Read the model definition and answer for the solid it produces. Units are mm, in the model's axes. Coordinates: 2 decimals unless noted, no trailing zeros. Write each loop counter-clockwise with the first axis right and the second up, starting at its lowest first coordinate (ties: lowest second). Pieces come first, ordered by that corner, then holes.
(1) Given pin 1 (6.5 mm diameter, centred on y = 8, z = 299, fed in from -X); pin 2 (4 mm diameter, centred on x = 314.5, y = 8.5, fed in from +Z); pin 3 (5 mm diameter, centred on y = 7.5, z = 7.5, fed in from -X), each flat-ended and moving along its own axis, determine where each tip first touches the part or whether it passes through.
(2) Section C-C on z = 265.5 is taken. Write down the section's boundary in (x, y).
(3) Section A-A on z = 37 is taken. Write down the section's boundary in (x, y), then the cut area to 3 significant figures.
(4) Find the intervals of material crossed by probe 1 along X at (y, z) = (1.5, -307.5); probe 2 along Z at (x, y) = (-57.5, 7.5); probe 3 along Z at (x, y) = (46, 6.25), in increasing order.
(5) The mould has two halves that part along Z. Classify faces 1 (the cylindrical face through (-253.76, 6.26, -11.08)), 2 (the flat face through (234, 12.7, -103)), 3 (the cylindrical face through (76.975, 6.261, -332.519)): +Z half, -Z half, draft (parallel to the pull), parting line (faces both ways), or undercut.
(6) Section B-B on x = -170 is taken. Write down the section's boundary in (y, z), then the cut area to 3 significant figures.
from build123d import *

# Parameters (mm, degrees)
BOSS_EXTRUDE1_DEPTH                          = 12.7
M8X1_25_TAPPED_HOLE1_FOR_LOWERING_D          = 6.8
M8_CLEARANCE_HOLE1_FOR_SPACER_BLOCK_D        = 9
M8_CLEARANCE_HOLE2_FOR_CLAMP_TIGHTENIN_D     = 9
M8_CLEARANCE_HOLE2_FOR_CLAMP_TIGHTENIN_DEPTH = 20
M8X1_25_TAPPED_HOLE2_FOR_CLAMP_TIGHTEN_D     = 6.8
BOSS_EXTRUDE2_START                          = -12.7
BOSS_EXTRUDE2_HANDLES_DEPTH                  = 12.7


with BuildPart() as part:
    # Sketch1 → Boss-Extrude1 (new body)
    with BuildSketch(Plane(origin=(0, 0, 0), x_dir=(1, 0, 0), z_dir=(0, 1, 0))):
        with BuildLine():
            Line((275.144331903, 6), (253.92912397, 6))
            ThreePointArc((253.92912397, 6), (-254, 0), (253.92912397, -6))
            Line((253.92912397, -6), (275.067203981, -6))
            Line((275.067203981, -6), (336.321934193, -6))
            Line((336.321934193, -6), (336.321934193, -26))
            Line((336.321934193, -26), (286.321934193, -26))
            ThreePointArc((286.321934193, -26), (-287.5, 0), (286.321934193, 26))
            Line((286.321934193, 26), (336.321934193, 26))
            Line((336.321934193, 26), (336.321934193, 6))
            Line((336.321934193, 6), (275.144331903, 6))
        make_face()
    extrude(amount=BOSS_EXTRUDE1_DEPTH)

    # M8x1.25 Tapped Hole1 - For Lowering (through all)
    with Locations(Plane(origin=(0, 12.7, 0), x_dir=(1, 0, 0), z_dir=(0, 1, 0))):
        with Locations((135.375, -234.476378075), (-270.75, 0), (135.375, 234.476378075)):
            Hole(M8X1_25_TAPPED_HOLE1_FOR_LOWERING_D / 2)

    # M8 Clearance Hole1 - For Spacer Block (through all)
    with Locations(Plane(origin=(0, 12.7, 0), x_dir=(1, 0, 0), z_dir=(0, 1, 0))):
        with Locations((0, 270.75), (234.476378075, -135.375), (-234.476378075, -135.375)):
            Hole(M8_CLEARANCE_HOLE1_FOR_SPACER_BLOCK_D / 2)

    # M8 Clearance Hole2 - For Clamp Tightening
    with Locations(Plane(origin=(0, 0, -26), x_dir=(-1, 0, 0), z_dir=(0, 0, -1))):
        with Locations((-311.321934193, 6.35)):
            Hole(M8_CLEARANCE_HOLE2_FOR_CLAMP_TIGHTENIN_D / 2, depth=M8_CLEARANCE_HOLE2_FOR_CLAMP_TIGHTENIN_DEPTH)

    # M8x1.25 Tapped Hole2 - For Clamp Tightening (through all)
    with Locations(Plane.XY.offset(26)):
        with Locations((311.321934193, 6.35)):
            Hole(M8X1_25_TAPPED_HOLE2_FOR_CLAMP_TIGHTEN_D / 2)

    # Sketch14 → Boss-Extrude2 - Handles (add)
    with BuildSketch(Plane(origin=(0, 12.7, 0), x_dir=(1, 0, 0), z_dir=(0, 1, 0)).offset(BOSS_EXTRUDE2_START)):
        with BuildLine():
            Line((-52.5, 342.5), (52.5, 342.5))
            ThreePointArc((52.5, 342.5), (77.248737342, 332.248737342), (87.5, 307.5))
            Line((87.5, 307.5), (87.5, 273.861278753))
            ThreePointArc((87.5, 273.861278753), (75.076192149, 277.524441036), (62.5, 280.624304008))
            Line((62.5, 280.624304008), (62.5, 307.5))
            ThreePointArc((62.5, 307.5), (59.571067812, 314.571067812), (52.5, 317.5))
            Line((52.5, 317.5), (-52.5, 317.5))
            ThreePointArc((-52.5, 317.5), (-59.571067812, 314.571067812), (-62.5, 307.5))
            Line((-62.5, 307.5), (-62.5, 280.624304008))
            ThreePointArc((-62.5, 280.624304008), (-75.076192149, 277.524441036), (-87.5, 273.861278753))
            Line((-87.5, 273.861278753), (-87.5, 307.5))
            ThreePointArc((-87.5, 307.5), (-77.248737342, 332.248737342), (-52.5, 342.5))
        make_face()
    boss_extrude2_handles = extrude(amount=BOSS_EXTRUDE2_HANDLES_DEPTH)

    # Mirror1: Boss-Extrude2 - Handles across plane
    add(boss_extrude2_handles.mirror(Plane.XY))


solid = part.part
Response:
1. pin 1: stops at x = -87.5
1. pin 2: stops at z = 26
1. pin 3: stops at x = -287.46
2. outline: (-110.3, 0) - (110.3, 0) - (110.3, 12.7) - (-110.3, 12.7) - close
3. outline: (-285.11, 0) - (-251.29, 0) - (-251.29, 12.7) - (-285.11, 12.7) - close; (251.29, 0) - (285.11, 0) - (285.11, 12.7) - (251.29, 12.7) - close
3. area: 859 mm2
4. probe 1: x = -87.5 to -62.5, 62.5 to 87.5
4. probe 2: z = -342.14 to -316.16, -281.69 to -247.41, 247.41 to 281.69, 316.16 to 342.14
4. probe 3: z = -342.5 to -317.5, -283.8 to -249.8, 249.8 to 283.8, 317.5 to 342.5
5. face 1: undercut
5. face 2: draft
5. face 3: -Z half
6. outline: (0, -231.85) - (12.7, -231.85) - (12.7, -188.72) - (0, -188.72) - close; (0, 188.72) - (12.7, 188.72) - (12.7, 231.85) - (0, 231.85) - close
6. area: 1,100 mm2
